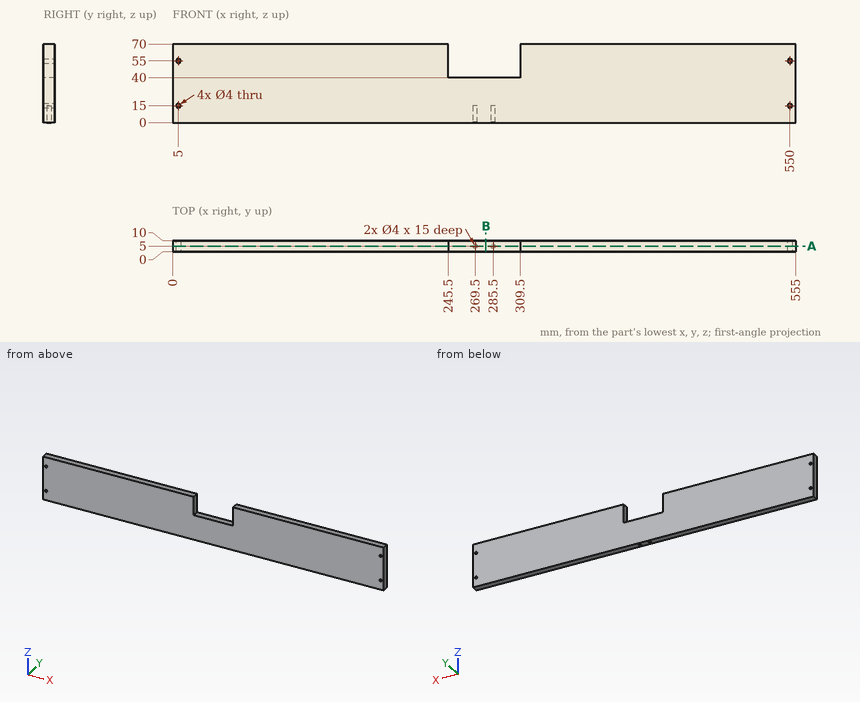
Drawing for the job (mm, zero at the part's lowest x, y, z). Give positions to 0.01 mm unless a question says otherwise; leave off trailing zeros. Order: outer loops, then holes, each group sorted by start corner. A loop starts at its lowest first (then second) coordinate and runs counter-clockwise, first axis right, second up. Notation, with made-up numbers: (-11.75, -29) -> (27.25, -29) arc R17 cw to (27.25, -8) -> close; hole circle Ø9 at (-8, -15). An arc over 180 degrees is marked (long way). Use one line per item in the form item = value.
(1) Saw through at A-A (y = 5). Write the cut outline in (x, z).
Solution:
outline = (0, 0) -> (267.5, 0) -> (267.5, 15) -> (271.5, 15) -> (271.5, 0) -> (283.5, 0) -> (283.5, 15) -> (287.5, 15) -> (287.5, 0) -> (555, 0) -> (555, 70) -> (309.5, 70) -> (309.5, 40) -> (245.5, 40) -> (245.5, 70) -> (0, 70) -> close; hole circle Ø4 at (5, 15); hole circle Ø4 at (5, 55); hole circle Ø4 at (550, 15); hole circle Ø4 at (550, 55)
(2) Flat gauge pins, fed straight in: P1, Ø5, axis at x = 289.5, y = 6.5, coming from the +Z side; P2, Ø1.2, axis at x = 286, y = 5.5, coming from the -Z side. Where does each tip first touch, or does it go through?
Solution:
P1 = 40
P2 = 15
(3) Saw through at B-B (x = 279). Write the cut outline in (y, z), then the cut area to 3 significant figures.
Solution:
outline = (0, 0) -> (10, 0) -> (10, 40) -> (0, 40) -> close
area = 400 mm²
(4) Drill centre lines: line 1 (X direction, y = 5, z = 11.5); line 2 (Y direction, x = 269.5, z = 5.5); line 3 (X direction, y = 4.25, z = 46.5). Where is each one in solid material? Low to high. Write a range as from..to.
Solution:
line_1 = 0..267.5, 271.5..283.5, 287.5..555
line_2 = 0..3, 7..10
line_3 = 0..245.5, 309.5..555
